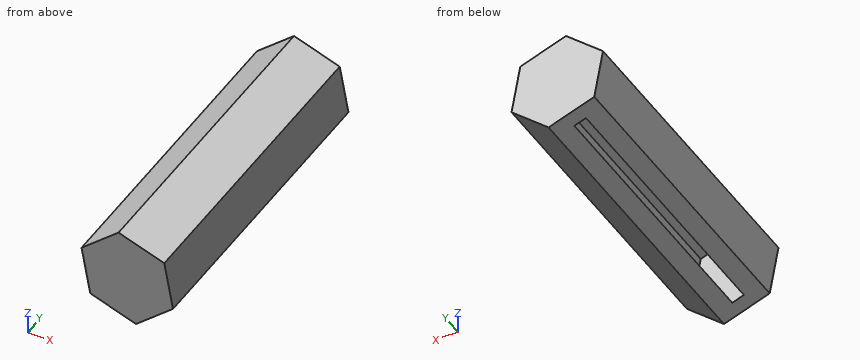
```python
from build123d import *

# Parameters (mm, degrees)
F1_DEPTH = 508
F2_T     = -25.4


with BuildPart() as f1:
    # F0 (on Front) → F1 (new body)
    with BuildSketch(Plane.XZ):
        Polygon((-58.7216, 38.701411), (-44.555271, -38.701411), (29.560703, -65.13442), (89.510348, -14.164609), (75.344019, 63.238212), (1.228045, 89.671222), align=None)
    extrude(amount=F1_DEPTH)

    # F2
    f2_openings = [f1.faces().sort_by_distance(p)[0] for p in [
        (-7.497284, -254, -51.917915),
    ]]
    offset(amount=F2_T, openings=f2_openings)


solid = f1.part
```
For this review, take the finished solid that the model builds, in its own axes (mm). Round coordinates to 2 decimals unless told otherwise and drop trailing zeros. Order: outer loops, then holes, each group sorted by start corner. A loop starts at its lowest first (then second) coordinate and runs counter-clockwise, first axis right, second up. Notation, with made-up numbers: (57.5, 61.25) -> (97.5, 61.25) arc R13 ccw to (97.5, 85.25) -> close; hole circle Ø9 at (46, 22). An arc over 180 degrees is marked (long way). Use a Markdown table: item, result.
Item 1: Take a section at C-C (z = 52). State the section outline as (x, y) points, plus the area to 3 significant figures.
Resolved:
| item | result |
|---|---|
| outline | (-43.08, -508) -> (77.4, -508) -> (77.4, 0) -> (-43.08, 0) -> close; hole (-3.87, -482.6) -> (31.24, -482.6) -> (31.24, -25.4) -> (-3.87, -25.4) -> close |
| area | 45,200 mm² |
Item 2: Take a section at D-D (x = -3.5). State the section outline as (y, z) points.
Resolved:
| item | result |
|---|---|
| outline | (-508, -53.34) -> (-482.6, -53.34) -> (-482.6, 52.31) -> (-25.4, 52.31) -> (-25.4, -53.34) -> (0, -53.34) -> (0, 85.65) -> (-508, 85.65) -> close |
Item 3: Take a section at A-A (x = 43). State the section outline as (y, z) points.
Resolved:
| item | result |
|---|---|
| outline | (-508, -53.71) -> (0, -53.71) -> (0, 74.77) -> (-508, 74.77) -> close; hole (-482.6, -20.37) -> (-25.4, -20.37) -> (-25.4, 47.81) -> (-482.6, 47.81) -> close |
Item 4: Take a section at B-B (y = -352). State the section outline as (x, z) points.
Resolved:
| item | result |
|---|---|
| outline | (-58.72, 38.7) -> (-44.56, -38.7) -> (-16.93, -48.55) -> (-31.1, 28.85) -> (6.51, 60.82) -> (53, 44.24) -> (61.89, -4.31) -> (1.94, -55.28) -> (29.56, -65.13) -> (89.51, -14.16) -> (75.34, 63.24) -> (1.23, 89.67) -> close |
Item 5: For pin 1 (5 mm diameter, centred on x = -29.5, y = -137, fed in from +Z); pin 2 (2 mm diameter, centred on x = 68.5, y = -80.5, fed in from +Z); pin 3 (10 mm diameter, centred on x = 74, y = -370, fed in from +Z), all flat-tipped, find the tip position at first contact; note any pin that passes through.
Resolved:
| item | result |
|---|---|
| pin 1 | stops at z = 65.67 |
| pin 2 | stops at z = 66.04 |
| pin 3 | stops at z = 65.5 |
Item 6: For line 1 along Y through (x, z) = (-7, 42); line 2 along X through (y, z) = (-172.5, 11.5); line 3 along Z through (x, y) = (49.5, -170), list the stretches that pass through material, from the lowest coordinate up. Write a range as [from, to].
Resolved:
| item | result |
|---|---|
| line 1 | y = [-508, -482.6], [-25.4, 0] |
| line 2 | x = [-53.74, -27.92], [58.99, 84.81] |
| line 3 | z = [-48.18, -14.84], [45.49, 72.46] |
